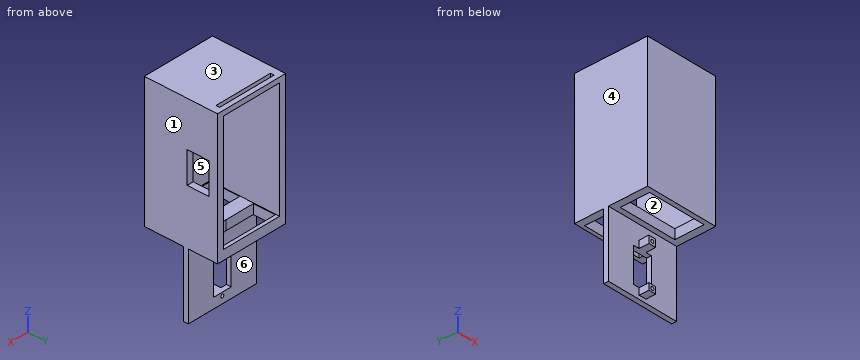
from build123d import *

# Parameters (mm, degrees)
SKETCH_1_W               = 50
SKETCH_1_H               = 50
EXTRUDE_1_DEPTH          = 80
EXTRUDE_1_DEPTH_BACK     = 55
SKETCH_2_W               = 41
SKETCH_2_H               = 80
CUT_EXTRUDE_1_DEPTH      = 47.5
SKETCH_3_W               = 13
SKETCH_3_H               = 23.5
CUT_EXTRUDE_2_DEPTH      = 60
CUT_EXTRUDE_2_DEPTH_BACK = 20
SKETCH_5_W               = 50
SKETCH_5_H               = 45
CUT_EXTRUDE_4_DEPTH      = 20
SKETCH_4_W               = 50
SKETCH_4_H               = 45
CUT_EXTRUDE_5_DEPTH      = 23
CUT_EXTRUDE_5_DEPTH_BACK = 10
CUT_EXTRUDE_6_DEPTH      = 10
SKETCH_7_W               = 40
SKETCH_7_H               = 20
CUT_EXTRUDE_7_DEPTH      = 10
SKETCH_9_W               = 40
SKETCH_9_H               = 2.5
CUT_EXTRUDE_8_DEPTH      = 10
SKETCH_11_W              = 5
SKETCH_11_H              = 4.5
SKETCH_11_H_2            = 5
EXTRUDE_4_DEPTH          = 10
SKETCH_13_W              = 21.5
SKETCH_13_H              = 15
CUT_EXTRUDE_10_DEPTH     = 15
SKETCH_14_R              = 1.1
CUT_EXTRUDE_11_DEPTH     = 12.4


with BuildPart() as part:
    # 草圖1 → 填料-伸長1 (new body, two sides)
    with BuildSketch(Plane.XY) as extrude_1_sk:
        with Locations((-3.62330355, 21.302402801)):
            Rectangle(SKETCH_1_W, SKETCH_1_H)
    extrude(amount=EXTRUDE_1_DEPTH)
    extrude(extrude_1_sk.sketch, amount=-EXTRUDE_1_DEPTH_BACK)

    # 草圖2 → 除料-伸長1 (cut)
    with BuildSketch(Plane(origin=(0, 46.302402801, 0), x_dir=(1, 0, 0), z_dir=(0, 1, 0))):
        with Locations((-3.62330355, -36.580275675)):
            Rectangle(SKETCH_2_W, SKETCH_2_H)
    extrude(amount=-CUT_EXTRUDE_1_DEPTH, mode=Mode.SUBTRACT)

    # 草圖3 → 除料-伸長2 (cut, two sides)
    with BuildSketch(Plane(origin=(0, 0, 0), x_dir=(1, 0, 0), z_dir=(0, 1, 0))) as cut_extrude_2_sk:
        with Locations((-3.62330355, 36.25)):
            Rectangle(SKETCH_3_W, SKETCH_3_H)
    extrude(amount=CUT_EXTRUDE_2_DEPTH, mode=Mode.SUBTRACT)
    extrude(cut_extrude_2_sk.sketch, amount=-CUT_EXTRUDE_2_DEPTH_BACK, mode=Mode.SUBTRACT)

    # 草圖5 → 除料-伸長4 (cut)
    with BuildSketch(Plane(origin=(0, 46.302402801, 0), x_dir=(1, 0, 0), z_dir=(0, 1, 0))):
        with Locations((-3.62330355, 32.5)):
            Rectangle(SKETCH_5_W, SKETCH_5_H)
    extrude(amount=-CUT_EXTRUDE_4_DEPTH, mode=Mode.SUBTRACT)

    # 草圖4 → 除料-伸長5 (cut, two sides)
    with BuildSketch(Plane(origin=(0, 0, 0), x_dir=(1, 0, 0), z_dir=(0, 1, 0))) as cut_extrude_5_sk:
        with Locations((-3.62330355, 32.5)):
            Rectangle(SKETCH_4_W, SKETCH_4_H)
    extrude(amount=CUT_EXTRUDE_5_DEPTH, mode=Mode.SUBTRACT)
    extrude(cut_extrude_5_sk.sketch, amount=-CUT_EXTRUDE_5_DEPTH_BACK, mode=Mode.SUBTRACT)

    # 草圖6 → 除料-伸長6 (cut)
    with BuildSketch(Plane(origin=(0, 0, -10), x_dir=(-1, 0, 0), z_dir=(0, 0, -1))):
        Polygon((3.693842319, 43.884561913), (-16.306157681, 43.884561913), (-16.306157681, 28.884561913), (3.67160538, 28.884561913), (23.649280632, 28.825329472), (23.693754411, 43.825263542), align=None)
    extrude(amount=-CUT_EXTRUDE_6_DEPTH, mode=Mode.SUBTRACT)

    # 草圖7 → 除料-伸長7 (cut)
    with BuildSketch(Plane(origin=(0, 0, -10), x_dir=(-1, 0, 0), z_dir=(0, 0, -1))):
        with Locations((3.768668362, 9.439500409)):
            Rectangle(SKETCH_7_W, SKETCH_7_H)
    extrude(amount=-CUT_EXTRUDE_7_DEPTH, mode=Mode.SUBTRACT)

    # 草圖9 → 除料-伸長8 (cut)
    with BuildSketch(Plane.XY.offset(80)):
        with Locations((-3.62330355, 41.816351076)):
            Rectangle(SKETCH_9_W, SKETCH_9_H)
    extrude(amount=-CUT_EXTRUDE_8_DEPTH, mode=Mode.SUBTRACT)

    # 草圖11 → 填料-伸長4 (add)
    with BuildSketch(Plane(origin=(0, 26.302402801, 0), x_dir=(1, 0, 0), z_dir=(0, 1, 0))):
        with Locations((-3.62330355, 50.25)):
            Rectangle(SKETCH_11_W, SKETCH_11_H)
        with Locations((-3.62330355, 22)):
            Rectangle(SKETCH_11_W, SKETCH_11_H_2)
    extrude(amount=-EXTRUDE_4_DEPTH)

    # 草圖13 → 除料-伸長10 (cut)
    with BuildSketch(Plane(origin=(21.37669645, 0, 0), x_dir=(0, 0, -1), z_dir=(1, 0, 0))):
        with Locations((-38.513161072, 32.983055623)):
            Rectangle(SKETCH_13_W, SKETCH_13_H)
    extrude(amount=-CUT_EXTRUDE_10_DEPTH, mode=Mode.SUBTRACT)

    # 草圖14 → 除料-伸長11 (cut)
    with BuildSketch(Plane(origin=(0, 26.302402801, 0), x_dir=(1, 0, 0), z_dir=(0, 1, 0))):
        with Locations((-3.62330355, 50.25)):
            Circle(SKETCH_14_R)
        with Locations((-3.62330355, 22)):
            Circle(SKETCH_14_R)
    extrude(amount=-CUT_EXTRUDE_11_DEPTH, mode=Mode.SUBTRACT)


solid = part.part
Source: CAD feature listing. Evaluate the final solid. Frame: model axes, mm. Face numbers are marked on the shaded views. A direction names the side the tool comes from. Give positions to 0.01 mm unless a question says otherwise; leave off trailing zeros. Write each loop counter-clockwise with the first axis right and the second up, starting at its lowest first coordinate (ties: lowest second). Pieces come first, ordered by that corner, then holes. Notation, with made-up numbers: M -15.75,48 L 31.25,48 A29 ccw 31.25,79 Z; hole C 62,30 d5. An arc over 180 degrees is marked long. Return JSON: item names as keys, results as strings. Group by question number.
1) Ray query, L1, parallel to Y at x = -6, z = -5.5; L2, parallel to Y at x = -19.5, z = -8.5; L3, parallel to X at y = 22, z = -22. Return the intervals inside material, ascending.
2) Draft query along Z for the marked faces 1, 2 and 3. Return one class per face: released by +Z, released by -Z, zero draft, split by the parting line, or undercut.
3) Cut plane B-B, the plane z = 13. Output: boundary loops of the cut face in (x, y).
4) First-contact query: pin 1 Ø5 at (y, z) = (18.5, -49.5) entering from +X; pin 2 Ø10 at (x, z) = (10.5, 37.5) entering from +Y; pin 3 Ø8 at (x, y) = (-14, 14.5) entering from -Z. Flat tips, straight axial feed; report the tip coordinate or a pass-through.
5) Cut plane A-A, the plane y = 11. Output: boundary loops of the cut face in (x, z), then the cut area to 3 significant figures.
6) Cut plane D-D, the plane z = -15. Output: boundary loops of the cut face in (x, y).
7) Cut plane C-C, the plane x = -18. Output: boundary loops of the cut face in (y, z), then the cut area to 3 significant figures.
8) Set-up query: the marked faces 4, 5 and 6. Return all of +Z, -Z, +X, -X, +Y, -Y with unobstructed straight access to the full face (end or side cutting, diameter ignored); none if empty.
Data:
{
 "1": {"L1": "y = -3.7 to -0.56, 19.44 to 28.88, 43.88 to 46.3", "L2": "y = -3.7 to -0.56, 19.44 to 28.84, 43.84 to 46.3", "L3": "x = -6.12 to -4.72, -2.52 to -1.12"},
 "2": {"face 1": "zero draft", "face 2": "undercut", "face 3": "released by +Z"},
 "3": {"outline": "M -28.62,-3.7 L 21.38,-3.7 L 21.38,46.3 L 16.88,46.3 L 16.88,-1.2 L -24.12,-1.2 L -24.12,46.3 L -28.62,46.3 Z"},
 "4": {"pin 1": "stops at x = -1.12", "pin 2": "stops at y = -1.2", "pin 3": "stops at z = 76.58"},
 "5": {"outline": "M -28.62,-10 L -23.77,-10 L -23.77,-3.42 L -24.12,-3.42 L -24.12,76.58 L 16.88,76.58 L 16.88,-3.42 L 16.23,-3.42 L 16.23,-10 L 21.38,-10 L 21.38,80 L -28.62,80 Z", "area": "957 mm²"},
 "6": {"outline": "M -28.62,23 L 21.38,23 L 21.38,26.3 L -28.62,26.3 Z"},
 "7": {"outline": "M -3.7,-10 L -0.56,-10 L -0.56,-3.42 L -1.2,-3.42 L -1.2,76.58 L 40.57,76.58 L 40.57,80 L -3.7,80 Z; M 19.44,-10 L 23,-10 L 23,-55 L 26.3,-55 L 26.3,-10 L 28.84,-10 L 28.84,-3.42 L 19.44,-3.42 Z; M 43.07,76.58 L 46.3,76.58 L 46.3,80 L 43.07,80 Z; M 43.84,-10 L 46.3,-10 L 46.3,-3.42 L 43.84,-3.42 Z", "area": "610 mm²"},
 "8": {"face 4": "+Z, -Z, -X, +Y, -Y", "face 5": "+Y", "face 6": "-Z, +X, -X, +Y"}
}
